The model under review builds one solid part; all positions refer to its coordinate system, in mm. Coordinates: 2 decimals unless noted, no trailing zeros. Order: outer loops, then holes, each group sorted by start corner. A loop starts at its lowest first (then second) coordinate and runs counter-clockwise, first axis right, second up. Notation, with made-up numbers: (6.25, 57.5) -> (24.25, 57.5) arc R12 cw to (24.25, 67.5) -> close; hole circle Ø4 at (-2.5, 42.25). An arc over 180 degrees is marked (long way). Use one line per item in the form item = value.
from build123d import *

# Parameters (mm, degrees)
F0_W     = 203
F0_H     = 403
F1_DEPTH = 3
F2_W     = 150
F2_H     = 300
F3_DEPTH = 25
F4_R     = 25
F5_W     = 203
F5_H     = 103
F6_DEPTH = 3


with BuildPart() as f1:
    # F0 (on Front) → F1 (new body)
    with BuildSketch(Plane.XZ):
        Rectangle(F0_W, F0_H)
    extrude(amount=F1_DEPTH)

    # F2 (on face) → F3 (cut)
    with BuildSketch(Plane.XZ.offset(3)):
        with Locations((26.5, 0)):
            Rectangle(F2_W, F2_H)
    extrude(amount=-F3_DEPTH, mode=Mode.SUBTRACT)

    # F4
    f4_edges = [f1.edges().sort_by_distance(p)[0] for p in [
        (-48.5, -1.5, 150),
        (-48.5, -1.5, -150),
    ]]
    fillet(f4_edges, radius=F4_R)

    # F5 (on face) → F6 (join, through all)
    with BuildSketch(Plane.XZ.offset(3)):
        with Locations((0, -253)):
            Rectangle(F5_W, F5_H)
    extrude(amount=-F6_DEPTH)


solid = f1.part
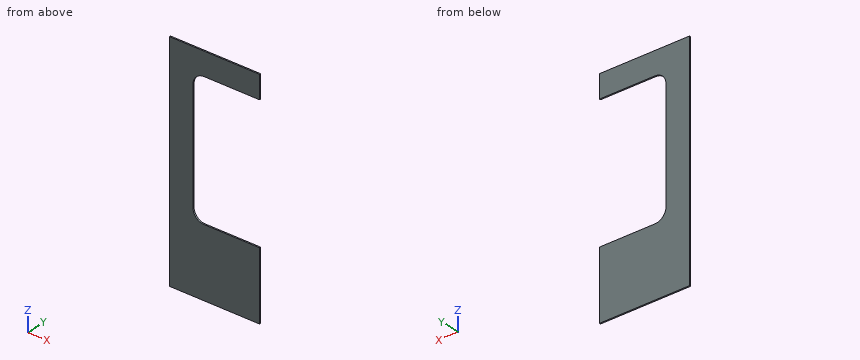
Item 1: Clearance check with a flat-ended pin moving along its axis: pin 1 (1.5 mm diameter, centred on y = -1.5, z = 24.5, fed in from +X). State where the tip first meets the part, or that it passes through.
Results found:
pin_1 = -48.5
Item 2: We need section A-A (x = -4). Write out the cut boundary in (y, z).
Results found:
outline = (-3, -304.5) -> (0, -304.5) -> (0, -150) -> (-3, -150) -> close; (-3, 150) -> (0, 150) -> (0, 201.5) -> (-3, 201.5) -> close
Item 3: We need section C-C (z = -73). Write out the cut boundary in (x, y), plus the area to 3 significant figures.
Results found:
outline = (-101.5, -3) -> (-48.5, -3) -> (-48.5, 0) -> (-101.5, 0) -> close
area = 159 mm²
Item 4: We need section B-B (y = -1). Write out the cut boundary in (x, z).
Results found:
outline = (-101.5, -304.5) -> (101.5, -304.5) -> (101.5, -150) -> (-23.5, -150) arc R25 cw to (-48.5, -125) -> (-48.5, 125) arc R25 cw to (-23.5, 150) -> (101.5, 150) -> (101.5, 201.5) -> (-101.5, 201.5) -> close
Item 5: To check wall thickness, follow L1, parallel to Z at x = 31, y = -0.95; L2, parallel to Z at x = -25.5, y = -0.2; L3, parallel to X at y = -1.8, z = -120.5. State the ranges of each line that lie inside material, in increasing order. Write a range as from..to.
Results found:
L1 = -304.5..-150, 150..201.5
L2 = -304.5..-149.92, 149.92..201.5
L3 = -101.5..-48.5
